Answer from the drawing. Dimensions are ordinates in mm from the lowest x, y and z of the part. Coordinates: 2 decimals unless noted, no trailing zeros. Order: outer loops, then holes, each group sorted by start corner. A loop starts at its lowest first (then second) coordinate and runs counter-clockwise, first axis right, second up. Notation, with made-up numbers: (83, 44.5) -> (124, 44.5) arc R22 ccw to (124, 62.5) -> close; hole circle Ø10 at (24.5, 29). An arc over 180 degrees is marked (long way). Answer in a Markdown table with one row per item.
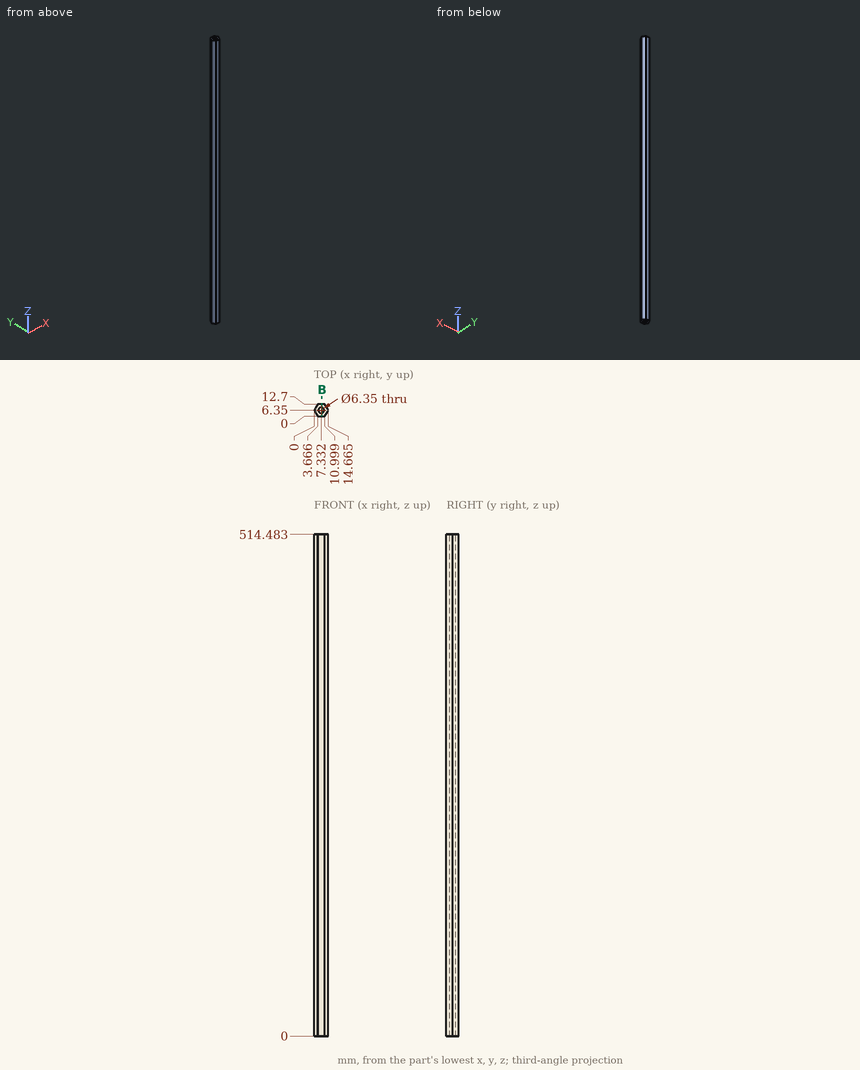
Q1. Consider line 1 (X direction, y = 9.25, z = 233.5) (1 decimal); line 2 (X direction, y = 7.5, z = 54) (1 decimal); line 3 (Y direction, x = 5.25, z = 341.5) (1 decimal). Determine where each line is inside the solid, lowest interval first.
Outcome:
| item | result |
|---|---|
| line 1 | 1.7 to 6, 8.6 to 13 |
| line 2 | 0.7 to 4.4, 10.3 to 14 |
| line 3 | 0 to 4, 8.7 to 12.7 |
Q2. Given pin 1 (1.5 mm diameter, centred on y = 6, z = 168.5, fed in from -X); pin 2 (1 mm diameter, centred on y = 8.5, z = 360, fed in from +X); pin 3 (4 mm diameter, centred on y = 3, z = 134.5, fed in from -X), each flat-ended and moving along its own axis, determine where each tip first touches the part or whether it passes through.
Outcome:
| item | result |
|---|---|
| pin 1 | x = 0 |
| pin 2 | x = 13.71 |
| pin 3 | x = 0.78 |
Q3. The part is cut by section B-B (x = 8). Write down the section's boundary in (y, z), then the cut area to 3 significant figures.
Outcome:
| item | result |
|---|---|
| outline | (0, 0) -> (3.25, 0) -> (3.25, 514.48) -> (0, 514.48) -> close; (9.45, 0) -> (12.7, 0) -> (12.7, 514.48) -> (9.45, 514.48) -> close |
| area | 3,340 mm² |
